Check sheet for the modelled part. Datum: model origin and axes. Units: mm. Face numbers are marked on the shaded views. A direction names the side the tool comes from. Round coordinates to 2 decimals unless told otherwise and drop trailing zeros. Write each loop counter-clockwise with the first axis right and the second up, starting at its lowest first coordinate (ties: lowest second). Pieces come first, ordered by that corner, then holes. Notation, with made-up numbers: (-4.5, 19.5) -> (39.5, 19.5) arc R20 cw to (39.5, 32.5) -> close; hole circle Ø4 at (77.5, 47). An arc over 180 degrees is marked (long way). Answer as a JSON object with one key per item and string values. Group by question number.
Autodesk Inventor part; units mm, degrees
ref_plane "YZ Plane" through (0, 0, 0) normal (1, 0, 0) x (0, 1, 0)
ref_plane "XZ Plane" through (0, 0, 0) normal (0, 1, 0) x (-1, 0, 0)
ref_plane "XY Plane" through (0, 0, 0) normal (0, 0, 1) x (1, 0, 0)
sketch "スケッチ1" plane through (0, 0, 0) normal (0, 1, 0) x (-1, 0, 0)
  circle A0 centre (0, 0) radius 2
  circle A1 centre (0, 0) radius 3.5
  circle A2 centre (0, 0) radius 4.25
  dimension "d0" = 4
  dimension "d1" = 7
  dimension "d2" = 8.5
extrude "押し出し1" add sketch "スケッチ1" along normal blind 2.5 contours A1
sketch "スケッチ2" plane through (0, 2.5, 0) normal (0, 1, 0) x (1, 0, 0)
  circle A0 centre (0, 0) radius 4.5
  dimension "d5" = 9
extrude "押し出し2" add sketch "スケッチ2" against normal blind 0.6
sketch "スケッチ3" plane through (0, 0, 0) normal (0, -1, 0) x (1, 0, 0)
  circle A0 centre (0, 0) radius 2
extrude "押し出し3" cut sketch "スケッチ3" against normal through all
sketch "スケッチ4" plane through (0, 2.5, 0) normal (0, 1, 0) x (1, 0, 0)
  circle A0 centre (0, 0) radius 4.5
  circle A1 centre (0, 0) radius 2.25
  circle A2 centre (0, 0) radius 3.25
  dimension "d10" = 4.5
  dimension "d11" = 6.5
extrude "押し出し4" cut sketch "スケッチ4" against normal blind 0.2 contours A2
sketch "スケッチ5" plane through (0, 0, 0) normal (0, -1, 0) x (1, 0, 0)
  circle A0 centre (0, 0) radius 2.25
  circle A1 centre (0, 0) radius 3.25
extrude "押し出し5" cut sketch "スケッチ5" against normal blind 0.2
properties part number "ベアリング3-7" material "アルミニウム 6061"
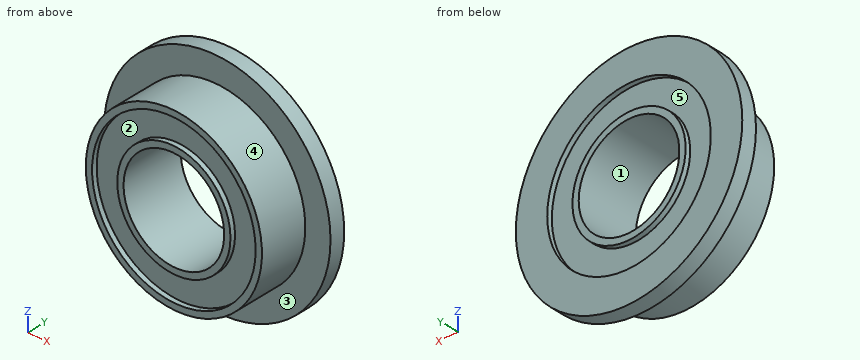
(1) Release check for a two-part mould opening along Z. For the marked faces 3, 4 and 5 record: pulls with the +Z half, pulls with the -Z half, needs draft (parallel to the pull), parting line crosses it, or undercut.
(2) Section check D-D on x = 2.5. Record the cut outline in (y, z), then the cut area to 3 significant figures.
(3) Section check A-A on x = 0. Record the cut outline in (y, z).
(4) Section check B-B on z = 0. Record the cut outline in (x, y), then the cut area to 3 significant figures.
(5) Section check C-C on y = 2.1. Record the cut outline in (x, z).
(6) Access from +Z, -Z, +X, -X, +Y, -Y to the whole of each face (thin tool, end or side, straight path). Record for the marked faces 1 and 2.
(7) Scan lines: line 1 along Z through (x, y) = (0, 2.4); line 2 along X through (y, z) = (0.7, 0). Record each from-to range of solid material in increasing order.
Data:
{
 "1": {"face 3": "needs draft", "face 4": "parting line crosses it", "face 5": "undercut"},
 "2": {"outline": "(0, -2.45) -> (1.9, -2.45) -> (1.9, -3.74) -> (2.5, -3.74) -> (2.5, -2.08) -> (2.3, -2.08) -> (2.3, 2.08) -> (2.5, 2.08) -> (2.5, 3.74) -> (1.9, 3.74) -> (1.9, 2.45) -> (0, 2.45) -> (0, 2.08) -> (0.2, 2.08) -> (0.2, -2.08) -> (0, -2.08) -> close", "area": "12.1 mm²"},
 "3": {"outline": "(0, -3.5) -> (1.9, -3.5) -> (1.9, -4.5) -> (2.5, -4.5) -> (2.5, -3.25) -> (2.3, -3.25) -> (2.3, -2.25) -> (2.5, -2.25) -> (2.5, -2) -> (0, -2) -> (0, -2.25) -> (0.2, -2.25) -> (0.2, -3.25) -> (0, -3.25) -> close; (0, 2) -> (2.5, 2) -> (2.5, 2.25) -> (2.3, 2.25) -> (2.3, 3.25) -> (2.5, 3.25) -> (2.5, 4.5) -> (1.9, 4.5) -> (1.9, 3.5) -> (0, 3.5) -> (0, 3.25) -> (0.2, 3.25) -> (0.2, 2.25) -> (0, 2.25) -> close"},
 "4": {"outline": "(-4.5, 1.9) -> (-3.5, 1.9) -> (-3.5, 0) -> (-3.25, 0) -> (-3.25, 0.2) -> (-2.25, 0.2) -> (-2.25, 0) -> (-2, 0) -> (-2, 2.5) -> (-2.25, 2.5) -> (-2.25, 2.3) -> (-3.25, 2.3) -> (-3.25, 2.5) -> (-4.5, 2.5) -> close; (2, 0) -> (2.25, 0) -> (2.25, 0.2) -> (3.25, 0.2) -> (3.25, 0) -> (3.5, 0) -> (3.5, 1.9) -> (4.5, 1.9) -> (4.5, 2.5) -> (3.25, 2.5) -> (3.25, 2.3) -> (2.25, 2.3) -> (2.25, 2.5) -> (2, 2.5) -> close", "area": "7.90 mm²"},
 "5": {"outline": "circle Ø9 at (0, 0); hole circle Ø4 at (0, 0)"},
 "6": {"face 1": "+Y, -Y", "face 2": "-Y"},
 "7": {"line 1": "z = -4.5 to -3.25, -2.25 to -2, 2 to 2.25, 3.25 to 4.5", "line 2": "x = -3.5 to -2, 2 to 3.5"}
}
